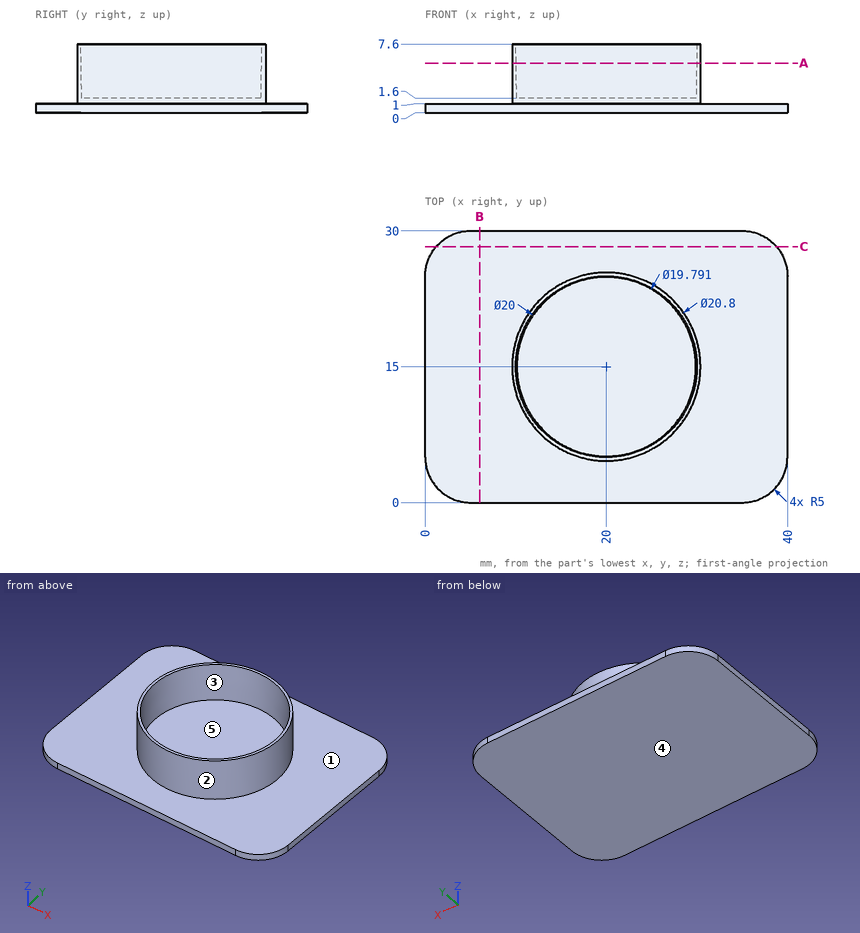
Answer from the drawing. Dimensions are ordinates in mm from the lowest x, y and z of the part. A direction names the side the tool comes from. Coordinates: 2 decimals unless noted, no trailing zeros. Write each loop counter-clockwise with the first axis right and the second up, starting at its lowest first coordinate (ties: lowest second). Pieces come first, ordered by that corner, then holes. Notation, with made-up numbers: (9, 59) - (53, 59) arc R32 cw to (53, 95) - close; hole circle Ø11 at (1.5, 27.25). An arc over 180 degrees is marked (long way). Answer as CSV lines item,"result".
1. Find section A-A (z = 5.5). Give the vertices of the cut face in (x, y).
Computed values:
outline,"circle Ø20.8 at (20, 15); hole circle Ø19.93 at (20, 15)"
2. Find section B-B (x = 6). Give the vertices of the cut face in (y, z).
Computed values:
outline,"(0, 0) - (30, 0) - (30, 1) - (0, 1) - close"
3. Straight lines are drawn through the part: line 1 (Z direction, x = 14, y = 14); line 2 (X direction, y = 9.25, z = 5.75) (1 decimal); line 3 (Y direction, x = 21.5, z = 3) (1 decimal). For each, find the intervals that lie inside material, in ascending order. Write a range as [from, to].
Computed values:
line 1,"z = [0, 1.6]"
line 2,"x = [11.3, 11.9], [28.1, 28.7]"
line 3,"y = [4.7, 5.2], [24.8, 25.3]"
4. Determine the mould class of the marked faces 1, 2 and 3 for opening direction X: +X half, -X half, draft (parallel to the pull), parting line (faces both ways), or undercut.
Computed values:
face 1,"draft"
face 2,"parting line"
face 3,"undercut"
5. A tool of negligible diameter and unlimited length cuts with its end or side. For the marked faces 4 and 5, from which of +Z, -Z, +X, -X, +Y, -Y can it reach the whole face along a straight path? Write none if from no direction.
Computed values:
face 4,"-Z, +X, -X, +Y, -Y"
face 5,"+Z"
6. Find section C-C (y = 28.25). Give the vertices of the cut face in (x, z).
Computed values:
outline,"(1.2, 0) - (38.8, 0) - (38.8, 1) - (1.2, 1) - close"
7. Given P1, Ø4, axis at y = 11.5, z = 4, coming from the +X side; P2, Ø4, axis at y = 14.5, z = 3.5, coming from the -X side; P3, Ø10, axis at x = 23, y = 22, coming from the +Z side; P4, Ø10, axis at x = 22.5, y = 16, coming from the +Z side, each flat-ended and moving along its own axis, determine where each tip first touches the part or whether it passes through.
Computed values:
P1,"stops at x = 30.29"
P2,"stops at x = 9.6"
P3,"stops at z = 7.6"
P4,"stops at z = 1.6"
